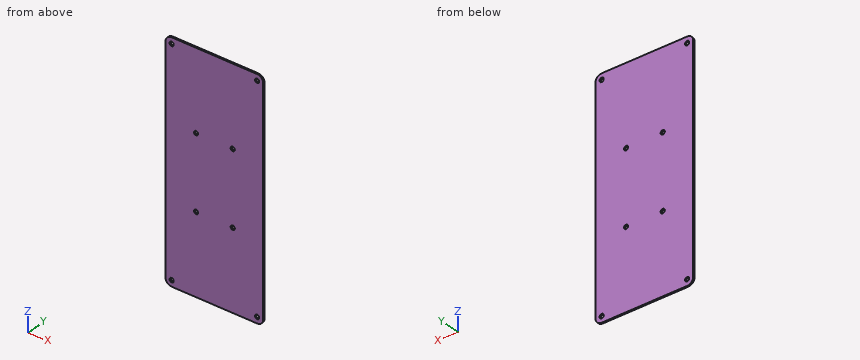
Autodesk Inventor part; units mm, degrees
ref_plane "YZ Plane" through (0, 0, 0) normal (1, 0, 0) x (0, 1, 0)
ref_plane "XZ Plane" through (0, 0, 0) normal (0, 1, 0) x (-1, 0, 0)
ref_plane "XY Plane" through (0, 0, 0) normal (0, 0, 1) x (1, 0, 0)
sketch "Sketch1" plane through (0, 0, 0) normal (0, 1, 0) x (-1, 0, 0)
  circle A0 centre (0, 0) radius 2.1844
  circle A1 centre (0, -228.6) radius 2.1844
  circle A2 centre (88.9, 0) radius 2.1844
  circle A3 centre (88.9, -228.6) radius 2.1844
  circle A4 centre (63.5, -76.2) radius 2.1844
  circle A5 centre (63.5, -152.4) radius 2.1844
  circle A6 centre (25.4, -152.4) radius 2.1844
  circle A7 centre (25.4, -76.2) radius 2.1844
  line L0 (95.25, 0) -> (95.25, -228.6)
  line L1 (88.9, -234.95) -> (0, -234.95)
  line L2 (-6.35, -228.6) -> (-6.35, 0)
  line L3 (0, 6.35) -> (88.9, 6.35)
  arc A8 (95.25, 0) -> (88.9, 6.35) centre (88.9, 0) ccw
  arc A9 (88.9, -234.95) -> (95.25, -228.6) centre (88.9, -228.6) ccw
  arc A10 (-6.35, -228.6) -> (0, -234.95) centre (0, -228.6) ccw
  arc A11 (0, 6.35) -> (-6.35, 0) centre (0, 0) ccw
  line L4 (88.9, 0) -> (88.9, -228.6)
  line L5 (0, 0) -> (0, -228.6)
  point P0 (44.45, -114.3)
  point P1 (44.45, -114.3)
  dimension "d0" = 4.3688
  dimension "d2" = 4.3688
  dimension "d7" = 4.3688
  dimension "d8" = 4.3688
  dimension "d15" = 4.3688
  dimension "d16" = 4.3688
  dimension "d17" = 4.3688
  dimension "d18" = 4.3688
extrude "Extrusion1" add sketch "Sketch1" along normal blind 1.5875
properties part number "brainmount(pocketlater)"
Geometry check sheet. Reference: the model listing, model coordinates, mm. Round coordinates to 2 decimals unless told otherwise and drop trailing zeros. Loops run counter-clockwise (first coordinate to the right, second up) from the corner with the lowest first, then second, coordinate; pieces in that order, holes last.
Item 1: Thickness scan on line 1 (X direction, y = 0.5, z = 0); line 2 (X direction, y = 0.5, z = -152.4); line 3 (Z direction, x = -61.5, y = 0.65). Record the ranges inside material, lowest first.
Item 2: Cross-section at A-A on x = -63.5. Record the boundary of the cut face in (y, z).
Item 3: Gauge pin test, flat end, axial feed: pin 1 (3.5 mm diameter, centred on x = -88.9, z = 0, fed in from +Y). Record the tip position at first contact, or that the pin passes through.
Item 4: Cross-section at B-B on z = -76.2. Record the boundary of the cut face in (x, y), then the cut area to 3 significant figures.
Answer sheet:
1. line 1: x = -95.25 to -91.08, -86.72 to -2.18, 2.18 to 6.35
1. line 2: x = -95.25 to -65.68, -61.32 to -27.58, -23.22 to 6.35
1. line 3: z = -234.95 to -153.28, -151.52 to -77.08, -75.32 to 6.35
2. outline: (0, -234.95) - (1.59, -234.95) - (1.59, -154.58) - (0, -154.58) - close; (0, -150.22) - (1.59, -150.22) - (1.59, -78.38) - (0, -78.38) - close; (0, -74.02) - (1.59, -74.02) - (1.59, 6.35) - (0, 6.35) - close
3. pin 1: passes through
4. outline: (-95.25, 0) - (-65.68, 0) - (-65.68, 1.59) - (-95.25, 1.59) - close; (-61.32, 0) - (-27.58, 0) - (-27.58, 1.59) - (-61.32, 1.59) - close; (-23.22, 0) - (6.35, 0) - (6.35, 1.59) - (-23.22, 1.59) - close
4. area: 147 mm2
